from build123d import *

# Parameters (mm, degrees)
SKETCH1_R           = 16
SKETCH1_R_2         = 7.5
BOSS_EXTRUDE1_DEPTH = 10
SKETCH1_3_R         = 16
SKETCH1_3_R_2       = 7.5
CUT_EXTRUDE1_DEPTH  = 6
SKETCH1_4_R         = 7.5
CUT_EXTRUDE2_DEPTH  = 10
CUT_EXTRUDE3_DEPTH  = 6
SKETCH3_R           = 1.75
CUT_EXTRUDE4_DEPTH  = 10
SKETCH4_R           = 3.25
CUT_EXTRUDE5_DEPTH  = 4


with BuildPart() as part:
    # Sketch1 → Boss-Extrude1 (new body)
    # profile 1 of 4: a face of its own
    with BuildSketch(Plane.XY):
        with BuildLine():
            ThreePointArc((-22, 9), (-19.084519704, 9.716037695), (-16.832454361, 11.701217039))
            ThreePointArc((-16.832454361, 11.701217039), (0, 20.5), (16.832454361, 11.701217039))
            ThreePointArc((16.832454361, 11.701217039), (19.084519704, 9.716037695), (22, 9))
            ThreePointArc((22, 9), (31, 0), (22, -9))
            ThreePointArc((22, -9), (19.084519704, -9.716037695), (16.832454361, -11.701217039))
            ThreePointArc((16.832454361, -11.701217039), (0, -20.5), (-16.832454361, -11.701217039))
            ThreePointArc((-16.832454361, -11.701217039), (-19.084519704, -9.716037695), (-22, -9))
            ThreePointArc((-22, -9), (-31, 0), (-22, 9))
        make_face()
        with BuildLine():
            ThreePointArc((-14.369168357, -9.988843813), (0, -17.5), (14.369168357, -9.988843813))
            ThreePointArc((14.369168357, -9.988843813), (17.694757076, -7.057361363), (22, -6))
            ThreePointArc((22, -6), (28, 0), (22, 6))
            ThreePointArc((22, 6), (17.694757076, 7.057361363), (14.369168357, 9.988843813))
            ThreePointArc((14.369168357, 9.988843813), (0, 17.5), (-14.369168357, 9.988843813))
            ThreePointArc((-14.369168357, 9.988843813), (-17.694757076, 7.057361363), (-22, 6))
            ThreePointArc((-22, 6), (-28, 0), (-22, -6))
            ThreePointArc((-22, -6), (-17.694757076, -7.057361363), (-14.369168357, -9.988843813))
        make_face(mode=Mode.SUBTRACT)
    # profile 2 of 4: a face of its own
    with BuildSketch(Plane.XY):
        with BuildLine():
            ThreePointArc((-22, -6), (-17.694757076, -7.057361363), (-14.369168357, -9.988843813))
            ThreePointArc((-14.369168357, -9.988843813), (0, -17.5), (14.369168357, -9.988843813))
            ThreePointArc((14.369168357, -9.988843813), (17.694757076, -7.057361363), (22, -6))
            ThreePointArc((22, -6), (28, 0), (22, 6))
            ThreePointArc((22, 6), (17.694757076, 7.057361363), (14.369168357, 9.988843813))
            ThreePointArc((14.369168357, 9.988843813), (0, 17.5), (-14.369168357, 9.988843813))
            ThreePointArc((-14.369168357, 9.988843813), (-17.694757076, 7.057361363), (-22, 6))
            ThreePointArc((-22, 6), (-28, 0), (-22, -6))
        make_face()
        Circle(SKETCH1_R, mode=Mode.SUBTRACT)
    # profile 3 of 4: a face of its own
    with BuildSketch(Plane.XY):
        Circle(SKETCH1_R)
        Circle(SKETCH1_R_2, mode=Mode.SUBTRACT)
    # profile 4 of 4: a face of its own
    with BuildSketch(Plane.XY):
        Circle(SKETCH1_R_2)
    extrude(amount=BOSS_EXTRUDE1_DEPTH)

    # Sketch1_3 → Cut-Extrude1 (cut)
    with BuildSketch(Plane.XY):
        Circle(SKETCH1_3_R)
        Circle(SKETCH1_3_R_2, mode=Mode.SUBTRACT)
    extrude(amount=CUT_EXTRUDE1_DEPTH, mode=Mode.SUBTRACT)

    # Sketch1_4 → Cut-Extrude2 (cut)
    with BuildSketch(Plane.XY):
        Circle(SKETCH1_4_R)
    extrude(amount=CUT_EXTRUDE2_DEPTH, mode=Mode.SUBTRACT)

    # Sketch1_5 → Cut-Extrude3 (cut)
    with BuildSketch(Plane.XY):
        with BuildLine():
            ThreePointArc((-22, 9), (-19.084519704, 9.716037695), (-16.832454361, 11.701217039))
            ThreePointArc((-16.832454361, 11.701217039), (0, 20.5), (16.832454361, 11.701217039))
            ThreePointArc((16.832454361, 11.701217039), (19.084519704, 9.716037695), (22, 9))
            ThreePointArc((22, 9), (31, 0), (22, -9))
            ThreePointArc((22, -9), (19.084519704, -9.716037695), (16.832454361, -11.701217039))
            ThreePointArc((16.832454361, -11.701217039), (0, -20.5), (-16.832454361, -11.701217039))
            ThreePointArc((-16.832454361, -11.701217039), (-19.084519704, -9.716037695), (-22, -9))
            ThreePointArc((-22, -9), (-31, 0), (-22, 9))
        make_face()
        with BuildLine():
            ThreePointArc((-14.369168357, -9.988843813), (0, -17.5), (14.369168357, -9.988843813))
            ThreePointArc((14.369168357, -9.988843813), (17.694757076, -7.057361363), (22, -6))
            ThreePointArc((22, -6), (28, 0), (22, 6))
            ThreePointArc((22, 6), (17.694757076, 7.057361363), (14.369168357, 9.988843813))
            ThreePointArc((14.369168357, 9.988843813), (0, 17.5), (-14.369168357, 9.988843813))
            ThreePointArc((-14.369168357, 9.988843813), (-17.694757076, 7.057361363), (-22, 6))
            ThreePointArc((-22, 6), (-28, 0), (-22, -6))
            ThreePointArc((-22, -6), (-17.694757076, -7.057361363), (-14.369168357, -9.988843813))
        make_face(mode=Mode.SUBTRACT)
    extrude(amount=CUT_EXTRUDE3_DEPTH, mode=Mode.SUBTRACT)

    # Sketch3 → Cut-Extrude4 (cut)
    with BuildSketch(Plane.XY.offset(10)):
        with Locations((22, 0)):
            Circle(SKETCH3_R)
        with Locations((-22, 0)):
            Circle(SKETCH3_R)
    extrude(amount=-CUT_EXTRUDE4_DEPTH, mode=Mode.SUBTRACT)

    # Sketch4 → Cut-Extrude5 (cut)
    with BuildSketch(Plane.XY.offset(10)):
        with Locations((22, 0)):
            Circle(SKETCH4_R)
        with Locations((-22, 0)):
            Circle(SKETCH4_R)
    extrude(amount=-CUT_EXTRUDE5_DEPTH, mode=Mode.SUBTRACT)


solid = part.part
Verification items for the finished model (mm, model axes). A direction names the side the tool comes from. Coordinates: 2 decimals unless noted, no trailing zeros. Order: outer loops, then holes, each group sorted by start corner. A loop starts at its lowest first (then second) coordinate and runs counter-clockwise, first axis right, second up. Notation, with made-up numbers: (6.5, 70.25) -> (22.5, 70.25) arc R31 cw to (22.5, 101.25) -> close; hole circle Ø4 at (-18.5, 38). An arc over 180 degrees is marked (long way). Put each result on its own line as item: value. Start each with the question number.
1. Cross-section at D-D, the plane x = -8.5. Record the boundary of the cut face in (y, z).
2. Go/stop test with flat-tipped pins: pin 1 Ø3 at (x, z) = (-1.5, 5.5) entering from +Y; pin 2 Ø3 at (x, z) = (-19, 6) entering from -Y; pin 3 Ø9 at (x, y) = (0, 0) entering from -Z; pin 4 Ø2 at (x, z) = (6, 7.5) entering from +Y. Record where each tip stops, or that it passes through.
3. Cross-section at C-C, the plane z = 8.5. Record the boundary of the cut face in (x, y).
4. Cross-section at B-B, the plane y = 0. Count the separate pieces of the cut face and the enclosed holes in it, then the cut area to 3 significant figures.
5. Mould release check, pull along Y, two halves, no side actions. Record for faces 4 (the cylindrical face through (-23.75, 0.08, 3.04)), 5 (the cylindrical face through (-0.28, 20.5, 7.97)), 6 (the cylindrical face through (31, 0, 8)): released by +Y, released by -Y, zero draft, split by the parting line, or undercut.
6. Cross-section at A-A, the plane x = 0. Record the boundary of the cut face in (y, z).
7. Material ranges on L1, parallel to Y at x = -22, z = 7.6; L2, parallel to Y at x = 0, z = 1.7; L3, parallel to X at y = -10, z = 5, recorded low to high. Write a range as [from, to].
8. Access from +Z, -Z, +X, -X, +Y, -Y to the whole of each face (thin tool, end or side, straight path). Record for faces 1 (the cylindrical face through (-17.75, -7.03, 2.96)), 2 (the cylindrical face through (28, 0, 3)), 3 (the flat face through (9.3, -15.1, 6)).
Computed:
1. outline: (-18.65, 6) -> (-15.3, 6) -> (-15.3, 0) -> (-13.56, 0) -> (-13.56, 6) -> (13.56, 6) -> (13.56, 0) -> (15.3, 0) -> (15.3, 6) -> (18.65, 6) -> (18.65, 10) -> (-18.65, 10) -> close
2. pin 1: y = 20.5
2. pin 2: y = -10.89
2. pin 3: through
2. pin 4: y = 19.88
3. outline: (-22, -9) arc R6.29 cw to (-16.83, -11.7) arc R20.5 ccw to (16.83, -11.7) arc R6.29 cw to (22, -9) arc R9 ccw to (22, 9) arc R6.29 cw to (16.83, 11.7) arc R20.5 ccw to (-16.83, 11.7) arc R6.29 cw to (-22, 9) arc R9 ccw to start; hole circle Ø6.5 at (-22, 0); hole circle Ø15 at (0, 0); hole circle Ø6.5 at (22, 0)
4. separate pieces: 4
4. enclosed holes: 0
4. area: 238 mm2
5. face 4: undercut
5. face 5: released by +Y
5. face 6: split by the parting line
6. outline: (-20.5, 6) -> (-17.5, 6) -> (-17.5, 0) -> (-16, 0) -> (-16, 6) -> (-7.5, 6) -> (-7.5, 10) -> (-20.5, 10) -> close; (7.5, 6) -> (16, 6) -> (16, 0) -> (17.5, 0) -> (17.5, 6) -> (20.5, 6) -> (20.5, 10) -> (7.5, 10) -> close
7. L1: [-9, -3.25], [3.25, 9]
7. L2: [-17.5, -16], [16, 17.5]
7. L3: [-14.36, -12.49], [12.49, 14.36]
8. face 1: -Z, -X, -Y
8. face 2: -Z, +X
8. face 3: -Z
